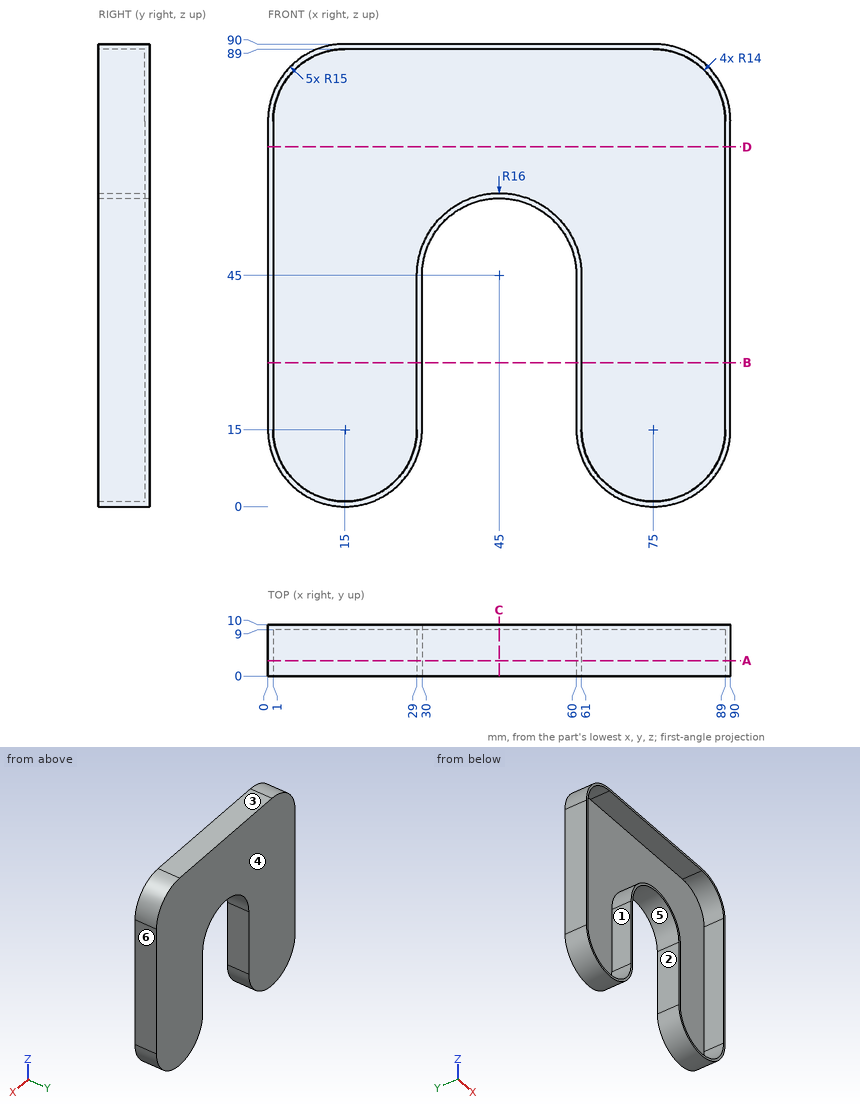
Study the drawing (mm; zero at the part's minimum x, y, z) and answer. A direction names the side the tool comes from. Coordinates: 2 decimals unless noted, no trailing zeros. Write each loop counter-clockwise with the first axis right and the second up, starting at its lowest first coordinate (ties: lowest second). Pieces come first, ordered by that corner, then holes.
Q1. Given P1, Ø1, axis at x = 80, z = 60.5, coming from the -Y side; P2, Ø1.5, axis at x = 27.5, y = 5, coming from the -Z side, each flat-ended and moving along its own axis, determine where each tip first touches the part or whether it passes through.
Returned:
P1: stops at y = 9
P2: stops at z = 5.68
Q2. Section A-A, the plane y = 3 is taken. Write down the section's boundary in (x, z).
Returned:
outline: (0, 15) arc R15 ccw to (30, 15) - (30, 45) arc R15 cw to (60, 45) - (60, 15) arc R15 ccw to (90, 15) - (90, 75) arc R15 ccw to (75, 90) - (15, 90) arc R15 ccw to (0, 75) - close; hole (1, 15) arc R14 ccw to (29, 15) - (29, 45) arc R16 cw to (61, 45) - (61, 15) arc R14 ccw to (89, 15) - (89, 75) arc R14 ccw to (75, 89) - (15, 89) arc R14 ccw to (1, 75) - close
Q3. Section B-B, the plane z = 28 is taken. Write down the section's boundary in (x, y), then the cut area to 3 significant figures.
Returned:
outline: (0, 0) - (1, 0) - (1, 9) - (29, 9) - (29, 0) - (30, 0) - (30, 10) - (0, 10) - close; (60, 0) - (61, 0) - (61, 9) - (89, 9) - (89, 0) - (90, 0) - (90, 10) - (60, 10) - close
area: 96.0 mm2
Q4. Which of the six approach directions +Z, -Z, +X, -X, +Y, -Y give full straight-line access (tool end or side, diameter ignored) to the marked faces 1, 2 and 3?
Returned:
face 1: -Y
face 2: -Z, +Y, -Y
face 3: +Z, +X, -X, +Y, -Y
Q5. The mould has two halves that part along X. Classify the marked faces 4, 5 and 6: released by +X, released by -X, zero draft, split by the parting line, or undercut.
Returned:
face 4: zero draft
face 5: undercut
face 6: released by +X
Q6. Section D-D, the plane z = 70 is taken. Write down the section's boundary in (x, y).
Returned:
outline: (0, 0) - (1, 0) - (1, 9) - (89, 9) - (89, 0) - (90, 0) - (90, 10) - (0, 10) - close
Q7. Find the intervals of material crossed by line 1 along X through (y, z) = (5.5, 29); line 2 along X through (y, z) = (2.5, 68.5); line 3 along X through (y, z) = (2.25, 50.5), in increasing order.
Returned:
line 1: x = 0 to 1, 29 to 30, 60 to 61, 89 to 90
line 2: x = 0 to 1, 89 to 90
line 3: x = 0 to 1, 29.98 to 31.04, 58.96 to 60.02, 89 to 90
Q8. Section C-C, the plane x = 45 is taken. Write down the section's boundary in (y, z).
Returned:
outline: (0, 60) - (10, 60) - (10, 90) - (0, 90) - (0, 89) - (9, 89) - (9, 61) - (0, 61) - close
